Geometry: final body of the model. Coordinates: model frame, mm. A direction names the side the tool comes from. Round coordinates to 2 decimals unless told otherwise and drop trailing zeros. Write each loop counter-clockwise with the first axis right and the second up, starting at its lowest first coordinate (ties: lowest second). Pieces come first, ordered by that corner, then holes. Notation, with made-up numbers: M 60,-36 L 103,-36 A14 cw 103,-9 Z; hole C 28,68 d7. An arc over 180 degrees is marked long. Put each result on its own line as item: value. Start each with the question number.
```python
from build123d import *

# Parameters (mm, degrees)
F2_R            = 9.9
F3_DEPTH        = 25
F5_DEPTH        = 25
F5_COPIES_COUNT = 23
F7_R            = 2.95
F8_DEPTH        = 24.9


# Not quite as in the source:
# - a feature of the source that left no trace in its solid (it failed there, or was rolled back) is left out
# - a pattern or mirror of a feature is missing from the dataset's text; its kind, count and spacing are read off the source's solid


with BuildPart() as f1:
    # F0 (on Front) → F1 (revolve)
    with BuildSketch(Plane.XZ):
        Polygon((0, 15.95), (0, 0), (20.2, 0), (20.2, 24.65), (10.2, 24.65), (10.2, 15.95), align=None)
    revolve(axis=Axis((10.1, 0, 0), (-1, 0, 0)))

    # F2 (on face) → F3 (cut)
    with BuildSketch(Plane(origin=(0, 0, 0), x_dir=(0, -1, 0), z_dir=(-1, 0, 0))):
        Circle(F2_R)
    extrude(amount=-F3_DEPTH, mode=Mode.SUBTRACT)

    # F4 (on face) → F5 (cut)
    with BuildSketch(Plane.YZ.offset(20.2)):
        with BuildLine():
            ThreePointArc((0.9605272399, 20.4764837905), (1.5385061373, 22.5929437067), (2.6011700561, 24.5123726787))
            ThreePointArc((2.6011700561, 24.5123726787), (0, 24.65), (-2.6011700561, 24.5123726787))
            ThreePointArc((-2.6011700561, 24.5123726787), (-1.5385061373, 22.5929437067), (-0.9605272399, 20.4764837905))
            ThreePointArc((-0.9605272399, 20.4764837905), (0, 20.499), (0.9605272399, 20.4764837905))
        make_face()
        with BuildLine():
            ThreePointArc((2.6011700561, 24.5123726787), (2.7312798677, 24.6882080288), (2.8655332609, 24.8609004137))
            ThreePointArc((2.8655332609, 24.8609004137), (0, 25.0255), (-2.8655332609, 24.8609004137))
            ThreePointArc((-2.8655332609, 24.8609004137), (-2.7312798677, 24.6882080288), (-2.6011700561, 24.5123726787))
            ThreePointArc((-2.6011700561, 24.5123726787), (0, 24.65), (2.6011700561, 24.5123726787))
        make_face()
    f5 = extrude(amount=-F5_DEPTH, mode=Mode.SUBTRACT)

    # F5_copies: F5 ×23 about axis
    f5_copies_axis = Axis((0, 0, 0), (1, 0, 0))
    for i in range(1, F5_COPIES_COUNT):
        add(f5.rotate(f5_copies_axis, i * 360 / F5_COPIES_COUNT), mode=Mode.SUBTRACT)

    # F7 (on Front) → F8 (cut, symmetric)
    with BuildSketch(Plane.XZ):
        with Locations((5.05, 0)):
            Circle(F7_R)
    extrude(amount=F8_DEPTH, both=True, mode=Mode.SUBTRACT)


solid = f1.part
```
1) Section C-C, the plane z = -9. Output: boundary loops of the cut face in (x, y), and give its area (3 significant figures).
2) Section A-A, the plane y = 0. Output: boundary loops of the cut face in (x, z).
3) Section B-B, the plane x = 5.05. Output: boundary loops of the cut face in (y, z).
4) Ray query, probe 1 along Z at (x, y) = (3.75, -0.5); probe 2 along Y at (x, z) = (17.75, -15.5); probe 3 along X at (y, z) = (-14.5, 0). Return the intervals inside material, ascending.
5) Section D-D, the plane z = 21.5. Output: boundary loops of the cut face in (x, y), and give its area (3 significant figures).
6) Draft query along Z for faces 1 (the face through (15.27, -2.78, -20.31)), 2 (the face through (15.27, 18.195, 9.443)), 3 (the face through (15.13, -15.565, 19.115)). Return one class per face: +Z half, -Z half, draft (parallel to the pull), parting line (faces both ways), or undercut.
7) First-contact query: pin 1 (4 mm diameter, centred on x = 16.5, z = 4, fed in from +Y); pin 2 (1 mm diameter, centred on x = 18, y = 15.5, fed in from +Z); pin 3 (1.5 mm diameter, centred on x = 15.5, z = -19, fed in from +Y); pin 4 (3.5 mm diameter, centred on x = 5.05, z = 0, fed in from -Y). Flat tips, straight axial feed; report the tip coordinate or a pass-through.
8) Access query for faces 4 (the face through (15.27, -17.587, -14.312)), 5 (the face through (15.27, -8.15, -18.81)), 6 (the face through (15.13, -23.23, 8.24)), 7 (the face through (15.27, 20.45, -1.39)), 8 (the face through (15.27, -1.55, 22.62)). Directions: +Z, -Z, +X, -X, +Y, -Y. A direction counts if a zero-diameter tool reaches every point of the face in a straight line with its end or side. Return the directions, or none.
Solved:
1. outline: M 0,-13.17 L 10.2,-13.17 L 10.2,-20.76 L 20.2,-20.76 L 20.2,-4.12 L 0,-4.12 Z; M 0,4.12 L 20.2,4.12 L 20.2,20.76 L 10.2,20.76 L 10.2,13.17 L 0,13.17 Z
1. area: 517 mm2
2. outline: M 0,-15.95 L 10.2,-15.95 L 10.2,-24.65 L 20.2,-24.65 L 20.2,-9.9 L 0,-9.9 Z; M 0,9.9 L 20.2,9.9 L 20.2,20.5 L 10.2,20.5 L 10.2,15.95 L 0,15.95 Z
3. outline: M -15.67,-2.95 A15.95 ccw 15.67,-2.95 L 9.45,-2.95 A9.9 cw -9.45,-2.95 Z; M -15.67,2.95 L -9.45,2.95 A9.9 cw 9.45,2.95 L 15.67,2.95 A15.95 ccw Z
4. probe 1: z = -15.94 to -9.89, 9.89 to 15.94
4. probe 2: y = -18.23 to -13.92, -13.41 to 13.41, 13.92 to 18.23
4. probe 3: x = 0 to 2.1, 8 to 20.2
5. outline: M 10.2,-10.54 L 20.2,-10.54 L 20.2,-7.7 L 10.2,-7.7 Z; M 10.2,-4.67 L 20.2,-4.67 L 20.2,-1.17 L 10.2,-1.17 Z; M 10.2,1.17 L 20.2,1.17 L 20.2,4.67 L 10.2,4.67 Z; M 10.2,7.7 L 20.2,7.7 L 20.2,10.54 L 10.2,10.54 Z
5. area: 127 mm2
6. face 1: -Z half
6. face 2: undercut
6. face 3: +Z half
7. pin 1: stops at y = 24.57
7. pin 2: stops at z = 19.56
7. pin 3: stops at y = 13.35
7. pin 4: passes through
8. face 4: +X, -X, -Y
8. face 5: +X, -X
8. face 6: +Z, +X, -X, -Y
8. face 7: +X, -X, +Y
8. face 8: +Z, +X, -X
